from build123d import *

# Parameters (mm, degrees)
CROQUIS1_W              = 50.8
CROQUIS1_H              = 25.4
CROQUIS1_W_2            = 47.8
CROQUIS1_H_2            = 22.4
SALIENTE_EXTRUIR1_DEPTH = 85
CROQUIS2_R              = 16
CORTAR_EXTRUIR1_DEPTH   = 26


with BuildPart() as part:
    # Croquis1 → Saliente-Extruir1 (new body)
    with BuildSketch(Plane.XY):
        Rectangle(CROQUIS1_W, CROQUIS1_H)
        Rectangle(CROQUIS1_W_2, CROQUIS1_H_2, mode=Mode.SUBTRACT)
    extrude(amount=SALIENTE_EXTRUIR1_DEPTH)

    # Croquis2 → Cortar-Extruir1 (cut)
    with BuildSketch(Plane(origin=(0, -12.7, 0), x_dir=(-1, 0, 0), z_dir=(0, -1, 0))):
        with Locations((0, -60)):
            Circle(CROQUIS2_R)
    extrude(amount=-CORTAR_EXTRUIR1_DEPTH, mode=Mode.SUBTRACT)


solid = part.part
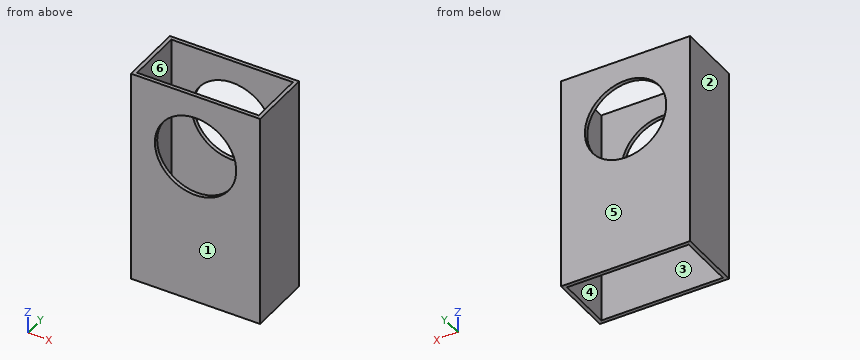
Could you check a few things on this model? Use its own coordinates, in mm. Face numbers are marked on the shaded views. A direction names the side the tool comes from. Give positions to 0.01 mm unless a question says otherwise; leave off trailing zeros. Loops run counter-clockwise (first coordinate to the right, second up) from the corner with the lowest first, then second, coordinate; pieces in that order, holes last. Notation, with made-up numbers: (-2.75, -35.75) -> (30.25, -35.75) arc R16 cw to (30.25, -21.75) -> close; hole circle Ø9 at (86.25, -34.75). An arc over 180 degrees is marked (long way). Return JSON: item names as keys, results as strings.
Item 1: We'd pull the mould along Y, two halves only. Please class the marked faces 1, 2, 3 and 4: +Y half, -Y half, draft (parallel to the pull), parting line (faces both ways), or undercut.
Geometry results:
{"face 1": "-Y half", "face 2": "draft", "face 3": "undercut", "face 4": "undercut"}
Item 2: If we section it at B-B on z = 60: List the corners of the cut face in (x, y) for me.
Geometry results:
{"outline": "(-25.4, -12.7) -> (-16, -12.7) -> (-16, -11.2) -> (-23.9, -11.2) -> (-23.9, 11.2) -> (-16, 11.2) -> (-16, 12.7) -> (-25.4, 12.7) -> close; (16, -12.7) -> (25.4, -12.7) -> (25.4, 12.7) -> (16, 12.7) -> (16, 11.2) -> (23.9, 11.2) -> (23.9, -11.2) -> (16, -11.2) -> close"}
Item 3: If we section it at A-A on x = 0: List the corners of the cut face in (y, z) for me.
Geometry results:
{"outline": "(-12.7, 0) -> (-11.2, 0) -> (-11.2, 44) -> (-12.7, 44) -> close; (-12.7, 76) -> (-11.2, 76) -> (-11.2, 85) -> (-12.7, 85) -> close; (11.2, 0) -> (12.7, 0) -> (12.7, 44) -> (11.2, 44) -> close; (11.2, 76) -> (12.7, 76) -> (12.7, 85) -> (11.2, 85) -> close"}
Item 4: If we section it at D-D on z = 25.5: List the corners of the cut face in (x, y) for me.
Geometry results:
{"outline": "(-25.4, -12.7) -> (25.4, -12.7) -> (25.4, 12.7) -> (-25.4, 12.7) -> close; hole (-23.9, -11.2) -> (23.9, -11.2) -> (23.9, 11.2) -> (-23.9, 11.2) -> close"}
Item 5: I'm going to push a flat-ended pin straight in: pin 1 (10 mm diameter, centred on x = -3, y = 9.5, fed in from +Z). Where does the tip first touch, or does it pass through?
Geometry results:
{"pin 1": "stops at z = 85"}
Item 6: Which directions (+Z, -Z, +X, -X, +Y, -Y) give clear straight access to the entire face, cutting with the end or side of a thin tool? Please do the marked faces 5 and 6.
Geometry results:
{"face 5": "+Z, -Z, +X, -X, +Y", "face 6": "+Z, -Z"}
Item 7: If we section it at C-C on y = -5.25: List the corners of the cut face in (x, z) for me.
Geometry results:
{"outline": "(-25.4, 0) -> (-23.9, 0) -> (-23.9, 85) -> (-25.4, 85) -> close; (23.9, 0) -> (25.4, 0) -> (25.4, 85) -> (23.9, 85) -> close"}
Item 8: I need wall thicknesses on L1, parallel to Y at x = 16.5, z = 35.5; L2, parallel to X at y = -12.35, z = 60; L3, parallel to X at y = 0.75, z = 35. Which ranges of each line are inside material? Lowest first, please. Write a range as from..to.
Geometry results:
{"L1": "y = -12.7..-11.2, 11.2..12.7", "L2": "x = -25.4..-16, 16..25.4", "L3": "x = -25.4..-23.9, 23.9..25.4"}
